The figure shows three views and two pictorial views of one solid part (mm, origin at its lowest corner). Answer the questions. A direction names the side the tool comes from. Round coordinates to 2 decimals unless told otherwise and drop trailing zeros. Order: outer loops, then holes, each group sorted by start corner. A loop starts at its lowest first (then second) coordinate and runs counter-clockwise, first axis right, second up. Notation, with made-up numbers: (-2, 15.25) - (50, 15.25) arc R22 cw to (50, 54.25) - close; hole circle Ø10 at (3, -2). An arc over 180 degrees is marked (long way). Answer in a Markdown table with one row per item.
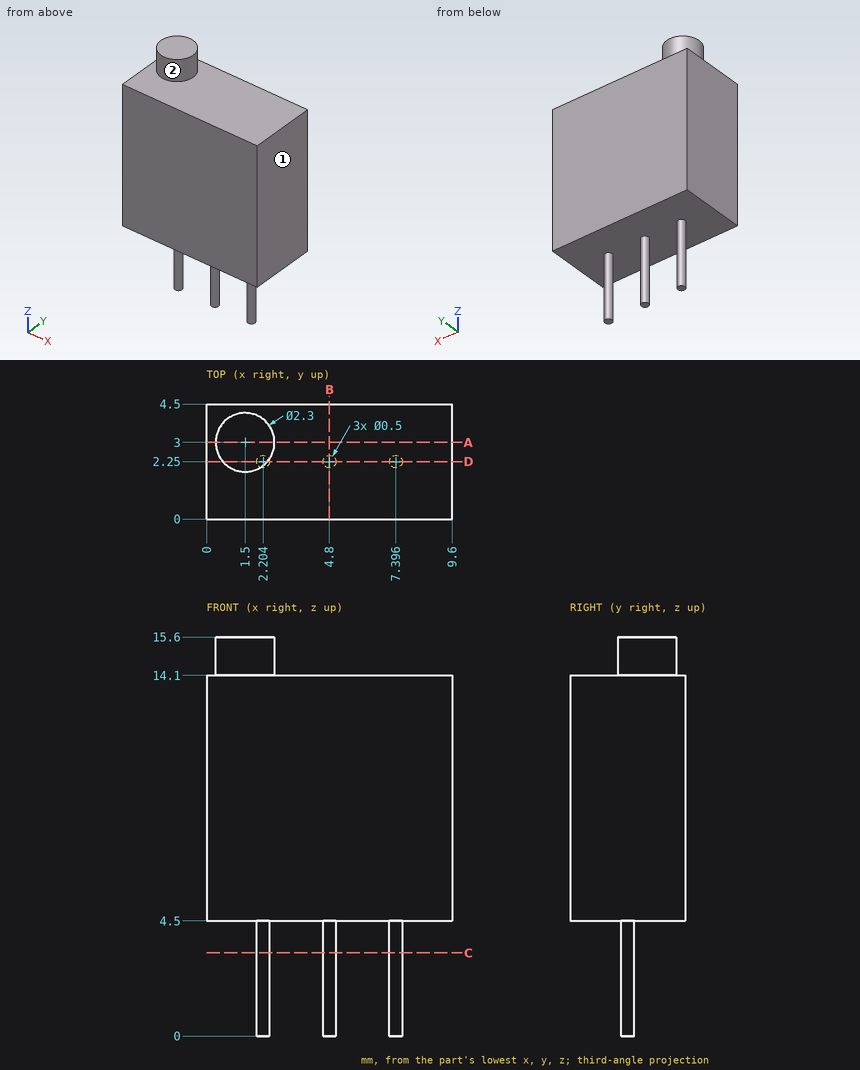
1) Find section A-A, the plane y = 3. Give the vertices of the cut face in (x, z).
Filled in:
| item | result |
|---|---|
| outline | (0, 4.5) - (9.6, 4.5) - (9.6, 14.1) - (2.65, 14.1) - (2.65, 15.6) - (0.35, 15.6) - (0.35, 14.1) - (0, 14.1) - close |
2) Find section B-B, the plane x = 4.8. Give the vertices of the cut face in (y, z), then the cut area to 4 significant figures.
Filled in:
| item | result |
|---|---|
| outline | (0, 4.5) - (2, 4.5) - (2, 0) - (2.5, 0) - (2.5, 4.5) - (4.5, 4.5) - (4.5, 14.1) - (0, 14.1) - close |
| area | 45.45 mm^2 |
3) Find the intervals of material crossed by probe 1 along Z at (x, y) = (4.25, 1.65); probe 2 along X at (y, z) = (2.05, 2); probe 3 along Z at (x, y) = (2, 2.95), in increasing order. Write a range as from..to.
Filled in:
| item | result |
|---|---|
| probe 1 | z = 4.5..14.1 |
| probe 2 | x = 2.05..2.35, 4.65..4.95, 7.25..7.55 |
| probe 3 | z = 4.5..15.6 |
4) Find section C-C, the plane z = 3.25. Give the vertices of the cut face in (x, y).
Filled in:
| item | result |
|---|---|
| outline | circle Ø0.5 at (2.2, 2.25); circle Ø0.5 at (4.8, 2.25); circle Ø0.5 at (7.4, 2.25) |
5) Which of the six approach directions +Z, -Z, +X, -X, +Y, -Y give full straight-line access (tool end or side, diameter ignored) to the marked faces 1 and 2?
Filled in:
| item | result |
|---|---|
| face 1 | +Z, -Z, +X, +Y, -Y |
| face 2 | +Z |
6) Find section D-D, the plane y = 2.25. Give the vertices of the cut face in (x, z).
Filled in:
| item | result |
|---|---|
| outline | (0, 4.5) - (1.95, 4.5) - (1.95, 0) - (2.45, 0) - (2.45, 4.5) - (4.55, 4.5) - (4.55, 0) - (5.05, 0) - (5.05, 4.5) - (7.15, 4.5) - (7.15, 0) - (7.65, 0) - (7.65, 4.5) - (9.6, 4.5) - (9.6, 14.1) - (2.37, 14.1) - (2.37, 15.6) - (0.63, 15.6) - (0.63, 14.1) - (0, 14.1) - close |
7) This flat-tipped pin is pushed along its axis until it touches: pin 1 (2 mm diameter, centred on x = 5, y = 2, fed in from -Z). Where does it stop, or does it pass through?
Filled in:
| item | result |
|---|---|
| pin 1 | stops at z = 0 |
